from build123d import *

# Parameters (mm, degrees)
F1_DEPTH = 20
F3_R     = 5
F3_W     = 13.5
F3_H     = 5.5
F4_DEPTH = 500
F6_W     = 33.5
F6_H     = 49.08588
F7_DEPTH = 10


with BuildPart() as f1:
    # F0 (on Right) → F1 (new body)
    with BuildSketch(Plane.YZ):
        Polygon((35.795717, 62), (0, 0), (46.188022, 0), (64.08588, 0), (81.983738, 31), (64.08588, 31), (81.983738, 62), align=None)
    extrude(amount=F1_DEPTH)

    # F3 (on face) → F4 (cut, symmetric)
    with BuildSketch(Plane(origin=(0, 16.02147, 27.75), x_dir=(1, 0, 0), z_dir=(0, -0.5, -0.866025))):
        with Locations((10, -10)):
            Circle(F3_R)
        with Locations((10, -30)):
            Circle(F3_R)
        with Locations((10, -47.75)):
            Rectangle(F3_W, F3_H)
    extrude(amount=F4_DEPTH, both=True, mode=Mode.SUBTRACT)

    # F5: F1 across plane


with BuildPart() as f1_1:
    add(f1.part)
    add(f1.part.mirror(Plane.YZ))

    # F6 (on face) → F7 (cut)
    with BuildSketch(Plane(origin=(0, 0, 0), x_dir=(1, 0, 0), z_dir=(0, 0, -1))):
        with Locations((0, -34.54294)):
            Rectangle(F6_W, F6_H)
    extrude(amount=-F7_DEPTH, mode=Mode.SUBTRACT)


solid = f1_1.part
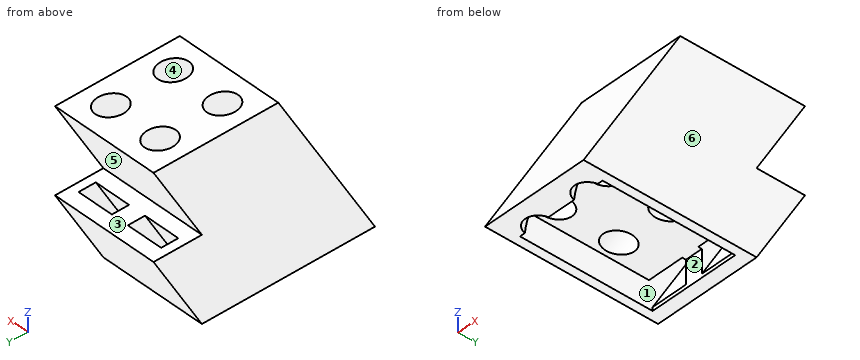
For this review, take the finished solid that the model builds, in its own axes (mm). Face numbers are marked on the shaded views. A direction names the side the tool comes from. Round coordinates to 2 decimals unless told otherwise and drop trailing zeros. Loops run counter-clockwise (first coordinate to the right, second up) from the corner with the lowest first, then second, coordinate; pieces in that order, holes last. Notation, with made-up numbers: (70, 64.5) - (110, 64.5) arc R29 cw to (110, 86.5) - close; hole circle Ø10 at (-23, 63.25). An arc over 180 degrees is marked (long way). Use one line per item in the form item = value.
Item 1: For line 1 (X direction, y = 60, z = 8); line 2 (Y direction, x = 14, z = 19.5); line 3 (X direction, y = 53, z = 32.5), list the stretches that pass through material, from the lowest coordinate up.
Answers:
line_1 = -20 to -16.75, -3.25 to 3.25, 16.75 to 20
line_2 = 11.26 to 19.34, 26.27 to 42.44, 49.36 to 63.22, 69.57 to 75.34
line_3 = -20 to -14.99, -5.01 to 5.01, 14.99 to 20
Item 2: Consider section A-A on x = 12. Write out the cut boundary in (y, z).
Answers:
outline = (0, 0) - (6.26, 0) - (10, 6.49) - (10, 10) - (12.03, 10) - (42.05, 62) - (35.8, 62) - close; (22.61, 10) - (35.12, 10) - (65.15, 62) - (52.63, 62) - close; (45.71, 10) - (57.74, 10) - (69.86, 31) - (64.09, 31) - (81.98, 62) - (75.73, 62) - close; (59.09, 0) - (64.09, 0) - (81.98, 31) - (76.21, 31) - (59.09, 1.34) - close
Item 3: Tool access review of the marked faces 1, 2 and 3: name each direction out of +Z, -Z, +X, -X, +Y, -Y from which nothing blocks a thin tool from reaching the whole face with its end or side.
Answers:
face_1 = none
face_2 = -Z
face_3 = +X, -X, +Y
Item 4: Consider section B-B on x = 0.5. Write out the cut boundary in (y, z).
Answers:
outline = (0, 0) - (10, 0) - (10, 10) - (59.09, 10) - (59.09, 0) - (64.09, 0) - (81.98, 31) - (64.09, 31) - (81.98, 62) - (35.8, 62) - close
Item 5: Consider section C-C on y = 49.5. State how many separate pieces and enclosed holes the cut face has, then the cut area to 3 significant figures.
Answers:
separate_pieces = 1
enclosed_holes = 2
area = 1,750 mm^2
Item 6: Mouldability with a two-part tool opening along X and no side actions: class the marked faces 4, 5 and 6 as +X half, -X half, draft (parallel to the pull), parting line (faces both ways), or undercut.
Answers:
face_4 = undercut
face_5 = draft
face_6 = +X half
Item 7: Consider section D-D on x = 7. Write out the cut boundary in (y, z), then the cut area to 3 significant figures.
Answers:
outline = (0, 0) - (6.93, 0) - (10, 5.32) - (10, 10) - (12.7, 10) - (42.72, 62) - (35.8, 62) - close; (21.94, 10) - (35.8, 10) - (65.82, 62) - (51.96, 62) - close; (45.03, 10) - (57.74, 10) - (69.86, 31) - (64.09, 31) - (81.98, 62) - (75.06, 62) - close; (59.09, 0) - (64.09, 0) - (81.98, 31) - (76.21, 31) - (59.09, 1.34) - close
area = 1,800 mm^2
Item 8: Clearance check with flat-ended pins moving along their axes: P1, Ø5, axis at x = -5, z = 3.5, coming from the +Y side; P2, Ø5, axis at x = -3, z = 7.5, coming from the -Y side; P3, Ø5, axis at x = 8.5, y = 48.5, coming from the +Z side. State where each tip first meets the part, or that it passes through.
Answers:
P1 = 67.55
P2 = 2.89
P3 = 59.5
